from build123d import *

# Parameters (mm, degrees)
F0_W     = 12.7
F0_H     = 11.0363
F2_R     = 2.54
F2_R_2   = 1.1176
F3_DEPTH = 30.43168


with BuildPart() as f1:
    # F0 (on Front) → F1 (revolve)
    with BuildSketch(Plane.XZ):
        with Locations((-6.876068, 2.367642)):
            Rectangle(F0_W, F0_H)
    revolve(axis=Axis((-6.876068, 0, -3.150508), (-1, 0, 0)))

    # F2 (on face) → F3 (cut)
    with BuildSketch(Plane(origin=(-13.226068, 0, 0), x_dir=(0, -1, 0), z_dir=(-1, 0, 0))):
        with Locations((0, -3.150508)):
            Circle(F2_R)
        with Locations((-5.51815, -3.150508)):
            Circle(F2_R_2)
        with Locations((0, 2.367642)):
            Circle(F2_R_2)
        with Locations((5.51815, -3.150508)):
            Circle(F2_R_2)
        with Locations((0, -8.668658)):
            Circle(F2_R_2)
    extrude(amount=-F3_DEPTH, mode=Mode.SUBTRACT)


solid = f1.part
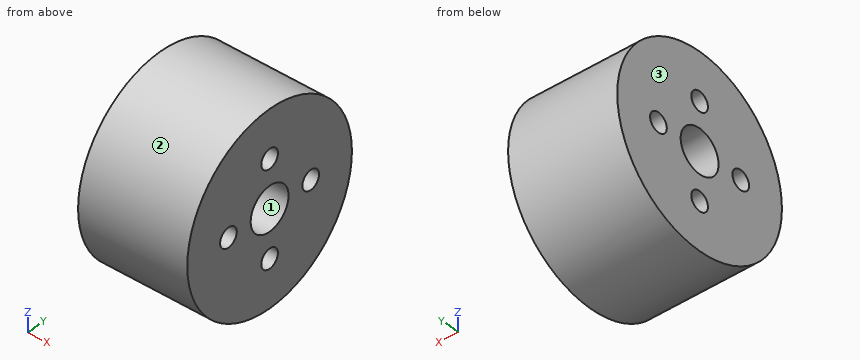
Check sheet for the modelled part. Datum: model origin and axes. Units: mm. Face numbers are marked on the shaded views. Give positions to 0.01 mm unless a question says otherwise; leave off trailing zeros. Write each loop counter-clockwise with the first axis right and the second up, starting at its lowest first coordinate (ties: lowest second). Pieces come first, ordered by that corner, then holes. Notation, with made-up numbers: M 12.25,81.5 L 25.25,81.5 A12 cw 25.25,97.5 Z; hole C 53,37 d7. An arc over 180 degrees is marked long. Use one line per item in the form item = value.
(1) Material ranges on line 1 along Z through (x, y) = (-8.75, 1); line 2 along Y through (x, z) = (-6, -4); line 3 along Z through (x, y) = (-8, -0.75), recorded low to high.
Answer block:
line_1 = -14.14 to -9.17, -8.17 to -5.49, -0.82 to 1.87, 2.87 to 7.84
line_2 = -11 to -6.24, -4.79 to -2.39, 2.39 to 4.79, 6.24 to 11
line_3 = -14.16 to -9.5, -7.84 to -5.58, -0.72 to 1.54, 3.2 to 7.86
(2) Depth check by flat-ended pin: P1, Ø6, axis at y = 0, z = -3.15, coming from the -X side. Enter the tip coordinate at first touch or a pass-through.
Answer block:
P1 = -13.23
(3) Section check B-B on z = 1.75. Record the boundary of the cut face in (x, y), plus the area to 3 significant figures.
Answer block:
outline = M -13.23,-9.89 L -0.53,-9.89 L -0.53,-0.93 L -13.23,-0.93 Z; M -13.23,0.93 L -0.53,0.93 L -0.53,9.89 L -13.23,9.89 Z
area = 228 mm2
(4) Section check D-D on z = 5. Record the boundary of the cut face in (x, y), plus the area to 3 significant figures.
Answer block:
outline = M -13.23,-7.44 L -0.53,-7.44 L -0.53,7.44 L -13.23,7.44 Z
area = 189 mm2
(5) Section check A-A on y = 0. Record the boundary of the cut face in (x, z).
Answer block:
outline = M -13.23,-14.19 L -0.53,-14.19 L -0.53,-9.79 L -13.23,-9.79 Z; M -13.23,-7.55 L -0.53,-7.55 L -0.53,-5.69 L -13.23,-5.69 Z; M -13.23,-0.61 L -0.53,-0.61 L -0.53,1.25 L -13.23,1.25 Z; M -13.23,3.49 L -0.53,3.49 L -0.53,7.89 L -13.23,7.89 Z
(6) Section check C-C on x = -3. Record the boundary of the cut face in (y, z), plus the area to 3 significant figures.
Answer block:
outline = C 0,-3.15 d22.07; hole C -5.52,-3.15 d2.24; hole C 0,-3.15 d5.08; hole C 0,-8.67 d2.24; hole C 0,2.37 d2.24; hole C 5.52,-3.15 d2.24
area = 347 mm2
(7) Draft check along Y on the marked faces 1, 2 and 3. Enter one of: pulls with the +Y half, pulls with the -Y half, needs draft (parallel to the pull), parting line crosses it, or undercut.
Answer block:
face_1 = undercut
face_2 = parting line crosses it
face_3 = needs draft
